Solid Edge part; units mm, degrees
sketch "Sketch1" plane through (0, 0, 0) normal (0, 0, 1) x (1, 0, 0)
  line L0 (-7.5, 0) -> (-7.5, 107.0096)
  arc A0 (-7.5, 107.0096) -> (7.5, 107.0096) centre (0, 120) cw
  line L1 (7.5, 107.0096) -> (7.5, 0)
  line L2 (7.5, 0) -> (-7.5, 0)
  circle A1 centre (-4, 116) radius 1
  circle A2 centre (4, 124) radius 1
  circle A3 centre (4, 116) radius 1
  circle A4 centre (-4, 124) radius 1
extrude "Protrusion1" add sketch "Sketch1" along normal blind 5.5
sketch "Sketch2" plane through (0, 70, 5.5) normal (0, 0, 1) x (0, -1, 0)
  line L0 (55, 7.5) -> (70, -7.5)
  line L1 (70, 7.5) -> (70, -7.5)
  line L2 (70, 7.5) -> (55, 7.5)
extrude "Cutout1" cut sketch "Sketch2" against normal through all
Geometry check sheet. Reference: the model listing, model coordinates, mm. A direction names the side the tool comes from. Round coordinates to 2 decimals unless told otherwise and drop trailing zeros. Loops run counter-clockwise (first coordinate to the right, second up) from the corner with the lowest first, then second, coordinate; pieces in that order, holes last. Notation, with made-up numbers: (71, 77.25) - (125, 77.25) arc R26 cw to (125, 92.25) - close; hole circle Ø2 at (79.5, 37.5). An arc over 180 degrees is marked (long way). Write item = value, one per line. Start each with the question number.
1. Section check C-C on x = -1.5. Enter the section's corners in (y, z), then the cut area to 3 significant figures.
2. Set-up check for faces 1 (the face through (7.5, 62, 3)), 2 (the face through (0, 83, 0)), 3 (the face through (-7.5, 53, 3)): record each of +Z, -Z, +X, -X, +Y, -Y from which the full face is reachable in a straight line by a thin tool's end or side.
3. Section check A-A on z = 4.3. Enter the section's corners in (x, y), then the cut area to 3 significant figures.
4. Depth check by flat-ended pin: pin 1 (3 mm diameter, centred on y = 111.5, z = 3, fed in from -X); pin 2 (1 mm diameter, centred on y = 103, z = 4, fed in from -X); pin 3 (1.5 mm diameter, centred on y = 66, z = 1, fed in from +X). Enter the tip coordinate at first touch or a pass-through.
5. Section check B-B on y = 103.5. Enter the section's corners in (x, z).
6. Thickness scan on line 1 (Y direction, x = -4, z = 4.15); line 2 (Y direction, x = 4.25, z = 3.35); line 3 (X direction, y = 116, z = 3). Record the ranges inside material, lowest first.
Working result:
q1.outline = (6, 0) - (134.92, 0) - (134.92, 5.5) - (6, 5.5) - close
q1.area = 709 mm^2
q2.face_1 = +Z, -Z, +X, -Y
q2.face_2 = -Z, +X, -X, +Y, -Y
q2.face_3 = +Z, -Z, -X, -Y
q3.outline = (-7.5, 0) - (7.5, 15) - (7.5, 107.01) arc R15 ccw (long way) to (-7.5, 107.01) - close; hole circle Ø2 at (-4, 116); hole circle Ø2 at (-4, 124); hole circle Ø2 at (4, 116); hole circle Ø2 at (4, 124)
q3.area = 2,170 mm^2
q4.pin_1 = -13.27
q4.pin_2 = -7.5
q4.pin_3 = 7.5
q5.outline = (-7.5, 0) - (7.5, 0) - (7.5, 5.5) - (-7.5, 5.5) - close
q6.line_1 = 3.5 to 115, 117 to 123, 125 to 134.46
q6.line_2 = 11.75 to 115.03, 116.97 to 123.03, 124.97 to 134.39
q6.line_3 = -14.46 to -5, -3 to 3, 5 to 14.46
